```python
from build123d import *

# Parameters (mm, degrees)
F1_DEPTH = 76.2
F2_DEPTH = 23.8125
F3_DEPTH = 50.8
F4_DEPTH = 63.5
F5_DEPTH = 25.4


# Not quite as in the source:
# - a feature names something its author has since deleted; it is built from what else it names


with BuildPart() as f1:
    # F0 (on Top) → F1 (new body)
    with BuildSketch(Plane.XY):
        with BuildLine():
            ThreePointArc((61.4074185531, -16.1672182717), (62.9746817305, -8.151040482), (63.5, 0))
            ThreePointArc((63.5, 0), (62.9746817305, 8.151040482), (61.4074185531, 16.1672182717))
            ThreePointArc((61.4074185531, 16.1672182717), (0, 63.5), (-61.4074185531, 16.1672182717))
            ThreePointArc((-61.4074185531, 16.1672182717), (-63.5, 0), (-61.4074185531, -16.1672182717))
            ThreePointArc((-61.4074185531, -16.1672182717), (0, -63.5), (61.4074185531, -16.1672182717))
        make_face()
        with BuildLine():
            ThreePointArc((26.9875, 46.7437211693), (42.8212465422, 32.8578981307), (52.135846474, 13.9697579594))
            ThreePointArc((52.135846474, 13.9697579594), (53.5132363927, 7.0451512251), (53.975, 0))
            ThreePointArc((53.975, 0), (53.5132363927, -7.0451512251), (52.135846474, -13.9697579594))
            ThreePointArc((52.135846474, -13.9697579594), (32.8578981307, -42.8212465422), (0, -53.975))
            ThreePointArc((0, -53.975), (-13.9697579594, -52.135846474), (-26.9875, -46.7437211693))
            ThreePointArc((-26.9875, -46.7437211693), (-42.8212465422, -32.8578981307), (-52.135846474, -13.9697579594))
            ThreePointArc((-52.135846474, -13.9697579594), (-53.975, 0), (-52.135846474, 13.9697579594))
            ThreePointArc((-52.135846474, 13.9697579594), (-32.8578981307, 42.8212465422), (0, 53.975))
            ThreePointArc((0, 53.975), (13.9697579594, 52.135846474), (26.9875, 46.7437211693))
        make_face(mode=Mode.SUBTRACT)
        with BuildLine():
            ThreePointArc((49.0690319755, 13.1480074912), (50.3653989578, 6.6307305648), (50.8, 0))
            ThreePointArc((50.8, 0), (50.3653989578, -6.6307305648), (49.0690319755, -13.1480074912))
            Line((49.0690319755, -13.1480074912), (52.135846474, -13.9697579594))
            ThreePointArc((52.135846474, -13.9697579594), (53.5132363927, -7.0451512251), (53.975, 0))
            ThreePointArc((53.975, 0), (53.5132363927, 7.0451512251), (52.135846474, 13.9697579594))
            Line((52.135846474, 13.9697579594), (49.0690319755, 13.1480074912))
        make_face()
        with BuildLine():
            ThreePointArc((25.4, 43.9940905122), (40.3023496868, 30.9250805936), (49.0690319755, 13.1480074912))
            Line((49.0690319755, 13.1480074912), (52.135846474, 13.9697579594))
            ThreePointArc((52.135846474, 13.9697579594), (42.8212465422, 32.8578981307), (26.9875, 46.7437211693))
            Line((26.9875, 46.7437211693), (25.4, 43.9940905122))
        make_face()
        with BuildLine():
            Line((52.135846474, -13.9697579594), (49.0690319755, -13.1480074912))
            ThreePointArc((49.0690319755, -13.1480074912), (30.9250805936, -40.3023496868), (0, -50.8))
            Line((0, -50.8), (0, -53.975))
            ThreePointArc((0, -53.975), (32.8578981307, -42.8212465422), (52.135846474, -13.9697579594))
        make_face()
        with BuildLine():
            ThreePointArc((0, 50.8), (13.1480074912, 49.0690319755), (25.4, 43.9940905122))
            Line((25.4, 43.9940905122), (26.9875, 46.7437211693))
            ThreePointArc((26.9875, 46.7437211693), (13.9697579594, 52.135846474), (0, 53.975))
            Line((0, 53.975), (0, 50.8))
        make_face()
        with BuildLine():
            Line((0, -53.975), (0, -50.8))
            ThreePointArc((0, -50.8), (-13.1480074912, -49.0690319755), (-25.4, -43.9940905122))
            Line((-25.4, -43.9940905122), (-26.9875, -46.7437211693))
            ThreePointArc((-26.9875, -46.7437211693), (-13.9697579594, -52.135846474), (0, -53.975))
        make_face()
        with BuildLine():
            ThreePointArc((-49.0690319755, 13.1480074912), (-30.9250805936, 40.3023496868), (0, 50.8))
            Line((0, 50.8), (0, 53.975))
            ThreePointArc((0, 53.975), (-32.8578981307, 42.8212465422), (-52.135846474, 13.9697579594))
            Line((-52.135846474, 13.9697579594), (-49.0690319755, 13.1480074912))
        make_face()
        with BuildLine():
            Line((-26.9875, -46.7437211693), (-25.4, -43.9940905122))
            ThreePointArc((-25.4, -43.9940905122), (-40.3023496868, -30.9250805936), (-49.0690319755, -13.1480074912))
            Line((-49.0690319755, -13.1480074912), (-52.135846474, -13.9697579594))
            ThreePointArc((-52.135846474, -13.9697579594), (-42.8212465422, -32.8578981307), (-26.9875, -46.7437211693))
        make_face()
        with BuildLine():
            ThreePointArc((-49.0690319755, -13.1480074912), (-50.8, 0), (-49.0690319755, 13.1480074912))
            Line((-49.0690319755, 13.1480074912), (-52.135846474, 13.9697579594))
            ThreePointArc((-52.135846474, 13.9697579594), (-53.975, 0), (-52.135846474, -13.9697579594))
            Line((-52.135846474, -13.9697579594), (-49.0690319755, -13.1480074912))
        make_face()
    extrude(amount=F1_DEPTH)

    # F0 (on Top) → F2 (join)
    with BuildSketch(Plane.XY):
        with BuildLine():
            ThreePointArc((-61.4074185531, -16.1672182717), (-63.5, 0), (-61.4074185531, 16.1672182717))
            Line((-61.4074185531, 16.1672182717), (-64.4777894091, 16.9755794573))
            ThreePointArc((-64.4777894091, 16.9755794573), (-66.675, 0), (-64.4777894091, -16.9755794573))
            Line((-64.4777894091, -16.9755794573), (-61.4074185531, -16.1672182717))
        make_face()
        with BuildLine():
            ThreePointArc((61.4074185531, 16.1672182717), (62.9746817305, 8.151040482), (63.5, 0))
            ThreePointArc((63.5, 0), (62.9746817305, -8.151040482), (61.4074185531, -16.1672182717))
            Line((61.4074185531, -16.1672182717), (64.4777894091, -16.9755794573))
            ThreePointArc((64.4777894091, -16.9755794573), (66.675, 0), (64.4777894091, 16.9755794573))
            Line((64.4777894091, 16.9755794573), (61.4074185531, 16.1672182717))
        make_face()
    extrude(amount=F2_DEPTH)

    # F0 (on Top) → F3 (cut)
    with BuildSketch(Plane.XY):
        with BuildLine():
            ThreePointArc((-49.0690319755, -13.1480074912), (-50.8, 0), (-49.0690319755, 13.1480074912))
            Line((-49.0690319755, 13.1480074912), (-52.135846474, 13.9697579594))
            ThreePointArc((-52.135846474, 13.9697579594), (-53.975, 0), (-52.135846474, -13.9697579594))
            Line((-52.135846474, -13.9697579594), (-49.0690319755, -13.1480074912))
        make_face()
        with BuildLine():
            ThreePointArc((49.0690319755, 13.1480074912), (50.3653989578, 6.6307305648), (50.8, 0))
            ThreePointArc((50.8, 0), (50.3653989578, -6.6307305648), (49.0690319755, -13.1480074912))
            Line((49.0690319755, -13.1480074912), (52.135846474, -13.9697579594))
            ThreePointArc((52.135846474, -13.9697579594), (53.5132363927, -7.0451512251), (53.975, 0))
            ThreePointArc((53.975, 0), (53.5132363927, 7.0451512251), (52.135846474, 13.9697579594))
            Line((52.135846474, 13.9697579594), (49.0690319755, 13.1480074912))
        make_face()
        with BuildLine():
            Line((-26.9875, -46.7437211693), (-25.4, -43.9940905122))
            ThreePointArc((-25.4, -43.9940905122), (-40.3023496868, -30.9250805936), (-49.0690319755, -13.1480074912))
            Line((-49.0690319755, -13.1480074912), (-52.135846474, -13.9697579594))
            ThreePointArc((-52.135846474, -13.9697579594), (-42.8212465422, -32.8578981307), (-26.9875, -46.7437211693))
        make_face()
        with BuildLine():
            ThreePointArc((25.4, 43.9940905122), (40.3023496868, 30.9250805936), (49.0690319755, 13.1480074912))
            Line((49.0690319755, 13.1480074912), (52.135846474, 13.9697579594))
            ThreePointArc((52.135846474, 13.9697579594), (42.8212465422, 32.8578981307), (26.9875, 46.7437211693))
            Line((26.9875, 46.7437211693), (25.4, 43.9940905122))
        make_face()
    extrude(amount=F3_DEPTH, mode=Mode.SUBTRACT)

    # F0 (on Top) → F4 (cut)
    with BuildSketch(Plane.XY):
        with BuildLine():
            Line((0, -53.975), (0, -50.8))
            ThreePointArc((0, -50.8), (-13.1480074912, -49.0690319755), (-25.4, -43.9940905122))
            Line((-25.4, -43.9940905122), (-26.9875, -46.7437211693))
            ThreePointArc((-26.9875, -46.7437211693), (-13.9697579594, -52.135846474), (0, -53.975))
        make_face()
        with BuildLine():
            ThreePointArc((0, 50.8), (13.1480074912, 49.0690319755), (25.4, 43.9940905122))
            Line((25.4, 43.9940905122), (26.9875, 46.7437211693))
            ThreePointArc((26.9875, 46.7437211693), (13.9697579594, 52.135846474), (0, 53.975))
            Line((0, 53.975), (0, 50.8))
        make_face()
    extrude(amount=F4_DEPTH, mode=Mode.SUBTRACT)

    # F0 (on Top) → F5 (join)
    with BuildSketch(Plane.XY):
        with BuildLine():
            Line((-26.9875, -46.7437211693), (-25.4, -43.9940905122))
            ThreePointArc((-25.4, -43.9940905122), (-40.3023496868, -30.9250805936), (-49.0690319755, -13.1480074912))
            Line((-49.0690319755, -13.1480074912), (-52.135846474, -13.9697579594))
            ThreePointArc((-52.135846474, -13.9697579594), (-42.8212465422, -32.8578981307), (-26.9875, -46.7437211693))
        make_face()
        with BuildLine():
            Line((0, -53.975), (0, -50.8))
            ThreePointArc((0, -50.8), (-13.1480074912, -49.0690319755), (-25.4, -43.9940905122))
            Line((-25.4, -43.9940905122), (-26.9875, -46.7437211693))
            ThreePointArc((-26.9875, -46.7437211693), (-13.9697579594, -52.135846474), (0, -53.975))
        make_face()
        with BuildLine():
            ThreePointArc((25.4, 43.9940905122), (40.3023496868, 30.9250805936), (49.0690319755, 13.1480074912))
            Line((49.0690319755, 13.1480074912), (52.135846474, 13.9697579594))
            ThreePointArc((52.135846474, 13.9697579594), (42.8212465422, 32.8578981307), (26.9875, 46.7437211693))
            Line((26.9875, 46.7437211693), (25.4, 43.9940905122))
        make_face()
        with BuildLine():
            ThreePointArc((0, 50.8), (13.1480074912, 49.0690319755), (25.4, 43.9940905122))
            Line((25.4, 43.9940905122), (26.9875, 46.7437211693))
            ThreePointArc((26.9875, 46.7437211693), (13.9697579594, 52.135846474), (0, 53.975))
            Line((0, 53.975), (0, 50.8))
        make_face()
    extrude(amount=F5_DEPTH)


solid = f1.part
```
The listing builds one solid part. Answer for the finished solid, in the listing's coordinates (mm). A direction names the side the tool comes from. Give positions to 0.01 mm unless a question says otherwise; leave off trailing zeros. Write each loop counter-clockwise with the first axis right and the second up, starting at its lowest first coordinate (ties: lowest second). Pieces come first, ordered by that corner, then holes. Notation, with made-up numbers: (78.5, 56.5) -> (111.5, 56.5) arc R28 cw to (111.5, 76.5) -> close; hole circle Ø2 at (-23.5, -18.5). An arc over 180 degrees is marked (long way). Write item = value, one per line. Start each with the question number.
1) The part is cut by section C-C, the plane x = 17. Determine the outline of the cut face in (y, z).
2) Each of these flat-tipped pins is pushed along its axis until it touches: pin 1 (3.5 mm diameter, centred on y = -52.5, z = 43.5, fed in from -X); pin 2 (12 mm diameter, centred on y = -24, z = 33.5, fed in from +X); pin 3 (2.5 mm diameter, centred on y = 52.5, z = 48, fed in from +X). Where does it stop, or does it pass through?
3) Straight lines are drawn through the part: line 1 along Z through (x, y) = (34, 40); line 2 along Y through (x, z) = (0, 20); line 3 along X through (y, z) = (47, 53). For each, find the intervals that lie inside material, in ascending order.
4) The part is cut by section B-B, the plane z = 16. Determine the outline of the cut face in (x, y) (3 decimals).
5) Which of the six approach directions +Z, -Z, +X, -X, +Y, -Y give full straight-line access (tool end or side, diameter ignored) to faces 1 (the face through (62.921, -16.566, 11.74)), 2 (the face through (50.581, 13.553, 12.522)), 3 (the face through (64, 0, 23.812)), 4 (the face through (62.964, 16.577, 11.74)), 5 (the face through (0, -52, 44))?
6) The part is cut by section A-A, the plane y = 24. Determine the outline of the cut face in (x, z).
7) Determine the mould class of faces 6 (the face through (-29, 43, 76.2)), 7 (the face through (13, 50, 63.5)), 8 (the face through (50.581, -13.553, 25.044)) for opening direction Z: +Z half, -Z half, draft (parallel to the pull), parting line (faces both ways), or undercut.
Solutions:
q1.outline = (-61.18, 0) -> (-47.87, 0) -> (-47.87, 76.2) -> (-61.18, 76.2) -> close; (47.87, 0) -> (61.18, 0) -> (61.18, 76.2) -> (47.87, 76.2) -> (47.87, 63.5) -> (51.23, 63.5) -> (51.23, 25.4) -> (47.87, 25.4) -> close
q2.pin_1 = -38.17
q2.pin_2 = 60.9
q2.pin_3 = 37.49
q3.line_1 = 0 to 25.4, 50.8 to 76.2
q3.line_2 = -63.5 to -50.8, 50.8 to 63.5
q3.line_3 = -42.7 to -19.28, 26.54 to 42.7
q4.outline = (-64.478, -16.976) -> (-61.407, -16.167) arc R63.5 ccw to (61.407, -16.167) -> (64.478, -16.976) arc R66.675 ccw to (64.478, 16.976) -> (61.407, 16.167) arc R63.5 ccw to (-61.407, 16.167) -> (-64.478, 16.976) arc R66.675 ccw to start; hole (-52.136, -13.97) -> (-49.069, -13.148) arc R50.8 ccw to (49.069, -13.148) -> (52.136, -13.97) arc R53.975 ccw to (52.136, 13.97) -> (49.069, 13.148) arc R50.8 ccw to (-49.069, 13.148) -> (-52.136, 13.97) arc R53.975 ccw to start
q5.face_1 = +Z, -Z, -Y
q5.face_2 = -Z
q5.face_3 = +Z, +X
q5.face_4 = +Z, -Z, +Y
q5.face_5 = none
q6.outline = (-58.79, 0) -> (-44.77, 0) -> (-44.77, 76.2) -> (-58.79, 76.2) -> close; (44.77, 0) -> (58.79, 0) -> (58.79, 76.2) -> (44.77, 76.2) -> (44.77, 50.8) -> (48.35, 50.8) -> (48.35, 25.4) -> (44.77, 25.4) -> close
q7.face_6 = +Z half
q7.face_7 = undercut
q7.face_8 = draft
